The model under review builds one solid part; all positions refer to its coordinate system, in mm. Face numbers are marked on the shaded views. A direction names the side the tool comes from. Coordinates: 2 decimals unless noted, no trailing zeros. Write each loop counter-clockwise with the first axis right and the second up, starting at its lowest first coordinate (ties: lowest second). Pieces come first, ordered by that corner, then holes. Notation, with made-up numbers: M -26,56.25 L 10,56.25 A27 cw 10,88.25 Z; hole C -39,63 d1. An arc over 180 degrees is marked long. Answer as a JSON object with one key per item and string values.
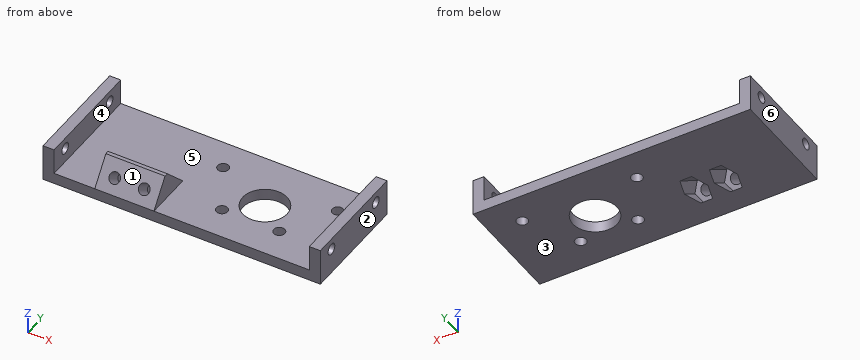
```python
from build123d import *

# Parameters (mm, degrees)
SKETCH1_W               = 75
SKETCH1_H               = 30
BOSS_EXTRUDE1_DEPTH     = 3
SKETCH2_W               = 3
SKETCH2_H               = 30
BOSS_EXTRUDE2_DEPTH     = 10
SKETCH4_R               = 1.5
CUT_EXTRUDE1_DEPTH      = 3
MIRROR1_COPY_1_SKETCH_R = 1.5
MIRROR1_COPY_1_DEPTH    = 3
SKETCH5_R               = 6
SKETCH5_R_2             = 1.5
CUT_EXTRUDE2_DEPTH      = 10
SKETCH6_W               = 16
SKETCH6_H               = 7
BOSS_EXTRUDE3_DEPTH     = 8
CHAMFER1_SIZE           = 7
CHAMFER1_SIZE2          = 5
SKETCH7_R               = 1.5
CUT_EXTRUDE3_DEPTH      = 5
CHAMFER2_SIZE           = 5
CHAMFER3_SIZE           = 2
CUT_EXTRUDE4_START      = -5
CUT_EXTRUDE4_DEPTH      = 42.544442581


with BuildPart() as part:
    # Sketch1 → Boss-Extrude1 (new body)
    with BuildSketch(Plane.XY):
        Rectangle(SKETCH1_W, SKETCH1_H)
    extrude(amount=BOSS_EXTRUDE1_DEPTH)

    # Sketch2 → Boss-Extrude2 (add)
    with BuildSketch(Plane(origin=(0, 0, 0), x_dir=(-1, 0, 0), z_dir=(0, 0, -1))):
        with Locations((-36, 0)):
            Rectangle(SKETCH2_W, SKETCH2_H)
    boss_extrude2 = extrude(amount=-BOSS_EXTRUDE2_DEPTH)

    # Sketch4 → Cut-Extrude1 (cut)
    with BuildSketch(Plane.ZY.offset(-34.5)):
        with Locations((7, 10)):
            Circle(SKETCH4_R)
    cut_extrude1 = extrude(amount=-CUT_EXTRUDE1_DEPTH, mode=Mode.SUBTRACT)

    # Mirror2: Cut-Extrude1 across plane
    add(cut_extrude1.mirror(Plane.ZX), mode=Mode.SUBTRACT)

    # Mirror1: Boss-Extrude2, Cut-Extrude1 across plane
    add(boss_extrude2.mirror(Plane(origin=(0, 0, 0), x_dir=(0, 0, 1), z_dir=(1, 0, 0))))
    add(cut_extrude1.mirror(Plane(origin=(0, 0, 0), x_dir=(0, 0, 1), z_dir=(1, 0, 0))), mode=Mode.SUBTRACT)

    # Mirror1 copy 1 sketch → Mirror1 copy 1 (cut)
    with BuildSketch(Plane(origin=(-34.5, 0, 0), x_dir=(0, 0, 1), z_dir=(1, 0, 0))):
        with Locations((7, 10)):
            Circle(MIRROR1_COPY_1_SKETCH_R)
    extrude(amount=-MIRROR1_COPY_1_DEPTH, mode=Mode.SUBTRACT)

    # Sketch5 → Cut-Extrude2 (cut)
    with BuildSketch(Plane.XY.offset(3)):
        with Locations((13.5, 0)):
            Circle(SKETCH5_R)
        with Locations((29, 7)):
            Circle(SKETCH5_R_2)
        with Locations((21.25, -6.423393759)):
            Circle(SKETCH5_R_2)
        with Locations((5.75, -6.423393759)):
            Circle(SKETCH5_R_2)
        with Locations((-2, 7)):
            Circle(SKETCH5_R_2)
    extrude(amount=-CUT_EXTRUDE2_DEPTH, mode=Mode.SUBTRACT)

    # Sketch6 → Boss-Extrude3 (add)
    with BuildSketch(Plane.XZ.offset(15)):
        with Locations((-15.5, 6.5)):
            Rectangle(SKETCH6_W, SKETCH6_H)
    extrude(amount=-BOSS_EXTRUDE3_DEPTH)

    # Chamfer1
    chamfer1_edges = [part.edges().sort_by_distance(p)[0] for p in [
        (-15.5, -15, 10),
    ]]
    chamfer1_side = [part.faces().sort_by_distance(p)[0] for p in [
        (0, -15, 0.756637298),
    ]]
    chamfer(chamfer1_edges, length=CHAMFER1_SIZE, length2=CHAMFER1_SIZE2, reference=chamfer1_side[0])

    # Sketch7 → Cut-Extrude3 (cut)
    with BuildSketch(Plane(origin=(0, -11.351351351, 8.108108108), x_dir=(1, 0, 0), z_dir=(0, -0.8137334712067348, 0.5812381937190968))):
        with Locations(Location((-19.5, -2.277372492, 0), (0, 0, 270))):
            Circle(SKETCH7_R)
        with Locations(Location((-11.5, -2.277372492, 0), (0, 0, 270))):
            Circle(SKETCH7_R)
    extrude(amount=-CUT_EXTRUDE3_DEPTH, mode=Mode.SUBTRACT)

    # Chamfer2
    chamfer2_edges = [part.edges().sort_by_distance(p)[0] for p in [
        (-15.5, -7, 3),
    ]]
    chamfer(chamfer2_edges, length=CHAMFER2_SIZE)

    # Chamfer3
    chamfer3_edges = [part.edges().sort_by_distance(p)[0] for p in [
        (-15.5, -7, 10),
    ]]
    chamfer(chamfer3_edges, length=CHAMFER3_SIZE - 0.0001)  # a hair under: the kernel refuses the full size

    # Sketch8 → Cut-Extrude4 (cut, through all)
    with BuildSketch(Plane(origin=(0, -11.351351351, 8.108108108), x_dir=(1, 0, 0), z_dir=(0, -0.8137334712067347, 0.5812381937190967)).offset(CUT_EXTRUDE4_START)):
        Polygon((-16.324573519, -2.277372492), (-17.91228676, 0.472627508), (-21.08771324, 0.472627508), (-22.675426481, -2.277372492), (-21.08771324, -5.027372492), (-17.91228676, -5.027372492), align=None)
        Polygon((-8.324573519, -2.277372492), (-9.91228676, 0.472627508), (-13.08771324, 0.472627508), (-14.675426481, -2.277372492), (-13.08771324, -5.027372492), (-9.91228676, -5.027372492), align=None)
    extrude(amount=-CUT_EXTRUDE4_DEPTH, mode=Mode.SUBTRACT)


solid = part.part
```
(1) Add section B-B on y = -3.25. Give the boundary of the cut face in (x, z).
Results list:
{"outline": "M -37.5,0 L -22.45,0 L -21.09,2.9 L -17.91,2.9 L -16.55,0 L -14.45,0 L -13.09,2.9 L -9.91,2.9 L -8.55,0 L 8.46,0 L 8.46,3 L -7.5,3 L -7.5,4.25 L -23.5,4.25 L -23.5,3 L -34.5,3 L -34.5,10 L -37.5,10 Z; M 18.54,0 L 37.5,0 L 37.5,10 L 34.5,10 L 34.5,3 L 18.54,3 Z"}
(2) Add section D-D on x = 32.5. Give the boundary of the cut face in (y, z), and give its area (3 significant figures).
Results list:
{"outline": "M -15,0 L 15,0 L 15,3 L -15,3 Z", "area": "90.0 mm²"}
(3) Add section C-C on x = 11. Give the boundary of the cut face in (y, z).
Results list:
{"outline": "M -15,0 L -5.45,0 L -5.45,3 L -15,3 Z; M 5.45,0 L 15,0 L 15,3 L 5.45,3 Z"}
(4) Add section A-A on x = 21.25. Give the boundary of the cut face in (y, z).
Results list:
{"outline": "M -15,0 L -7.92,0 L -7.92,3 L -15,3 Z; M -4.92,0 L 15,0 L 15,3 L -4.92,3 Z"}
(5) For pin 1 Ø9 at (x, y) = (-4, 5.5) entering from +Z; pin 2 Ø2.5 at (y, z) = (-10, 7) entering from +X; pin 3 Ø2 at (x, z) = (-11.5, 5.5) entering from +Y, all flat-tipped, find the tip position at first contact; note any pin that passes through.
Results list:
{"pin 1": "z = 3", "pin 2": "x = -7.5", "pin 3": "y = -3.5"}
(6) Wall thickness on line 1 along X through (y, z) = (0.5, 7); line 2 along Y through (x, z) = (36.7, 7); line 3 along X through (y, z) = (-9.75, 3.25): over which ranges is each line inside the solid? List them lowest first. Write a range as from..to.
Results list:
{"line 1": "-37.5..-34.5, 34.5..37.5", "line 2": "-15..-11.5, -8.5..8.5, 11.5..15", "line 3": "-37.5..-34.5, -23.5..-20.8, -18.2..-12.8, -10.2..-7.5, 34.5..37.5"}
(7) Draft analysis for pull direction X (two halves, no side actions). For the marked faces 1, 2 and 3, state which applies: released by +X, released by -X, zero draft, split by the parting line, or undercut.
Results list:
{"face 1": "undercut", "face 2": "released by +X", "face 3": "zero draft"}
(8) For the marked faces 4, 5 and 6, list the 3-axis set-ups (+Z, -Z, +X, -X, +Y, -Y) from which the entire face can be reached by the end or side of a thin tool; tool diameter is ignored.
Results list:
{"face 4": "+Z, +Y, -Y", "face 5": "+Z, +Y", "face 6": "+Z, -Z, -X, +Y, -Y"}
